The listing builds one solid part. Answer for the finished solid, in the listing's coordinates (mm). Face numbers are marked on the shaded views. Round coordinates to 2 decimals unless told otherwise and drop trailing zeros. Order: outer loops, then holes, each group sorted by start corner. A loop starts at its lowest first (then second) coordinate and runs counter-clockwise, first axis right, second up. Notation, with made-up numbers: (-7, -32.5) - (25, -32.5) arc R27 cw to (25, -12.5) - close; hole circle Ø10 at (80.25, 36). An arc over 180 degrees is marked (long way). Write item = value, one per line.
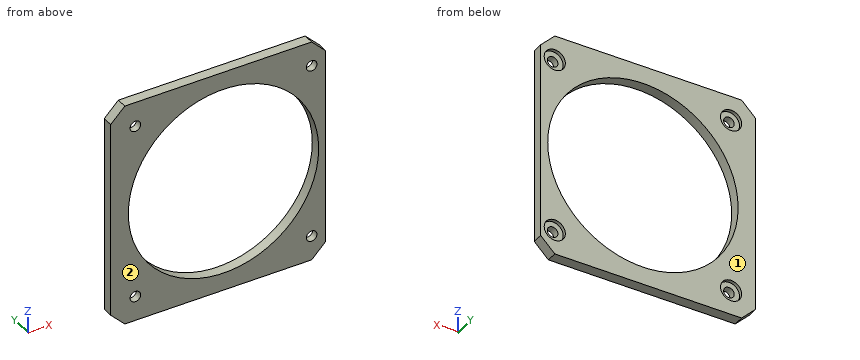
from build123d import *

# Parameters (mm, degrees)
CYLINDER871_R     = 3
CYLINDER871_DEPTH = 3
CYLINDER872_R     = 3
CYLINDER872_DEPTH = 3
CYLINDER873_R     = 3
CYLINDER873_DEPTH = 3
CYLINDER870_R     = 3
CYLINDER870_DEPTH = 3
CYLINDER867_R     = 27
CYLINDER867_DEPTH = 10
CYLINDER864_R     = 1.5
CYLINDER864_DEPTH = 10
CYLINDER865_R     = 1.5
CYLINDER865_DEPTH = 10
CYLINDER866_R     = 1.5
CYLINDER866_DEPTH = 10
CYLINDER863_R     = 1.5
CYLINDER863_DEPTH = 10
BOX418_W          = 61
BOX418_H          = 3
BOX418_DEPTH      = 64
CHAMFER023_SIZE   = 4
CHAMFER024_SIZE   = 4


with BuildPart() as obj1:
    # Cylinder871 → Cylinder871 (new body)
    with BuildSketch(Plane(origin=(50, 0, 0), x_dir=(1, 0, 0), z_dir=(0, -1, 0))):
        Circle(CYLINDER871_R)
    extrude(amount=CYLINDER871_DEPTH)


with BuildPart() as obj2:
    # Cylinder872 → Cylinder872 (new body)
    with BuildSketch(Plane(origin=(50, 0, 50), x_dir=(1, 0, 0), z_dir=(0, -1, 0))):
        Circle(CYLINDER872_R)
    extrude(amount=CYLINDER872_DEPTH)


with BuildPart() as obj3:
    # Cylinder873 → Cylinder873 (new body)
    with BuildSketch(Plane(origin=(0, 0, 50), x_dir=(1, 0, 0), z_dir=(0, -1, 0))):
        Circle(CYLINDER873_R)
    extrude(amount=CYLINDER873_DEPTH)


with BuildPart() as compound499:
    # Cylinder870 → Cylinder870 (new body)
    with BuildSketch(Plane.XZ):
        Circle(CYLINDER870_R)
    extrude(amount=CYLINDER870_DEPTH)

    # Compound499: union obj1, obj2, obj3
    add(obj1.part)
    add(obj2.part)
    add(obj3.part)


with BuildPart() as compound499_1:
    # Compound499 placement: moved
    add(compound499.part.moved(Location((7, 5, 7))))


with BuildPart() as obj4:
    # Cylinder867 → Cylinder867 (new body)
    with BuildSketch(Plane(origin=(32, 5, 32), x_dir=(1, 0, 0), z_dir=(0, -1, 0))):
        Circle(CYLINDER867_R)
    extrude(amount=CYLINDER867_DEPTH)


with BuildPart() as obj5:
    # Cylinder864 → Cylinder864 (new body)
    with BuildSketch(Plane(origin=(50, 0, 0), x_dir=(1, 0, 0), z_dir=(0, -1, 0))):
        Circle(CYLINDER864_R)
    extrude(amount=CYLINDER864_DEPTH)


with BuildPart() as obj6:
    # Cylinder865 → Cylinder865 (new body)
    with BuildSketch(Plane(origin=(50, 0, 50), x_dir=(1, 0, 0), z_dir=(0, -1, 0))):
        Circle(CYLINDER865_R)
    extrude(amount=CYLINDER865_DEPTH)


with BuildPart() as obj7:
    # Cylinder866 → Cylinder866 (new body)
    with BuildSketch(Plane(origin=(0, 0, 50), x_dir=(1, 0, 0), z_dir=(0, -1, 0))):
        Circle(CYLINDER866_R)
    extrude(amount=CYLINDER866_DEPTH)


with BuildPart() as compound498:
    # Cylinder863 → Cylinder863 (new body)
    with BuildSketch(Plane.XZ):
        Circle(CYLINDER863_R)
    extrude(amount=CYLINDER863_DEPTH)

    # Compound498: union obj5, obj6, obj7
    add(obj5.part)
    add(obj6.part)
    add(obj7.part)


with BuildPart() as compound498_1:
    # Compound498 placement: moved
    add(compound498.part.moved(Location((7, 4, 7))))


with BuildPart() as chamfer024:
    # Box418 → Box418 (new body)
    with BuildSketch(Plane.XY):
        with Locations((30.5, 1.5)):
            Rectangle(BOX418_W, BOX418_H)
    extrude(amount=BOX418_DEPTH)

    # Cut015: cut Compound498
    add(compound498_1.part, mode=Mode.SUBTRACT)

    # Cut016: cut obj4
    add(obj4.part, mode=Mode.SUBTRACT)

    # Cut019: cut Compound499
    add(compound499_1.part, mode=Mode.SUBTRACT)

    # Chamfer023
    chamfer023_edges = [chamfer024.edges().sort_by_distance(p)[0] for p in [
        (0, 1.5, 0),
        (61, 1.5, 0),
    ]]
    chamfer(chamfer023_edges, length=CHAMFER023_SIZE)

    # Chamfer024
    chamfer024_edges = [chamfer024.edges().sort_by_distance(p)[0] for p in [
        (0, 1.5, 64),
        (61, 1.5, 64),
    ]]
    chamfer(chamfer024_edges, length=CHAMFER024_SIZE)


solid = chamfer024.part
Q1. Section B-B on z = 32 is taken. Determine the outline of the cut face in (x, y), then the cut area to 3 significant figures.
Model answer:
outline = (0, 0) - (5, 0) - (5, 3) - (0, 3) - close; (59, 0) - (61, 0) - (61, 3) - (59, 3) - close
area = 21.0 mm^2
Q2. Section C-C on y = 2.5 is taken. Determine the outline of the cut face in (x, z).
Model answer:
outline = (0, 4) - (4, 0) - (57, 0) - (61, 4) - (61, 60) - (57, 64) - (4, 64) - (0, 60) - close; hole circle Ø6 at (7, 7); hole circle Ø6 at (7, 57); hole circle Ø54 at (32, 32); hole circle Ø6 at (57, 7); hole circle Ø6 at (57, 57)
Q3. Find the intervals of material crossed by line 1 (X direction, y = 2.55, z = 7); line 2 (X direction, y = 0.6, z = 7); line 3 (Z direction, x = 55, y = 2.25), in increasing order. Write a range as from..to.
Model answer:
line_1 = 0..4, 10..21.8, 42.2..54, 60..61
line_2 = 0..5.5, 8.5..21.8, 42.2..55.5, 58.5..61
line_3 = 0..4.76, 9.24..17.86, 46.14..54.76, 59.24..64
Q4. Section A-A on x = 32 is taken. Determine the outline of the cut face in (y, z), then the cut area to 3 significant figures.
Model answer:
outline = (0, 0) - (3, 0) - (3, 5) - (0, 5) - close; (0, 59) - (3, 59) - (3, 64) - (0, 64) - close
area = 30.0 mm^2
Q5. Determine the mould class of the marked faces 1 and 2 for opening direction Y: released by +Y, released by -Y, zero draft, split by the parting line, or undercut.
Model answer:
face_1 = released by +Y
face_2 = released by -Y
Q6. A flat-ended cylindrical pin translates along its axis: P1, Ø1.8, axis at x = 58.5, z = 7, coming from the +Y side. Find the tip coordinate at first contact, or state that the pin passes through.
Model answer:
P1 = 2
Q7. Section D-D on z = 57 is taken. Determine the outline of the cut face in (x, y), then the cut area to 3 significant figures.
Model answer:
outline = (0, 0) - (5.5, 0) - (5.5, 2) - (4, 2) - (4, 3) - (0, 3) - close; (8.5, 0) - (21.8, 0) - (21.8, 3) - (10, 3) - (10, 2) - (8.5, 2) - close; (42.2, 0) - (55.5, 0) - (55.5, 2) - (54, 2) - (54, 3) - (42.2, 3) - close; (58.5, 0) - (61, 0) - (61, 3) - (60, 3) - (60, 2) - (58.5, 2) - close
area = 97.8 mm^2
